```python
from build123d import *

# Parameters (mm, degrees)
SKETCH_W      = 45
SKETCH_H      = 161
PAD_DEPTH     = 10
SKETCH001_W   = 45
SKETCH001_H   = 10
PAD001_DEPTH  = 55.5
SKETCH002_R   = 2.75
HOLE_DEPTH    = 161.001
SKETCH003_W   = 45
SKETCH003_H   = 10
PAD002_DEPTH  = 45.4
SKETCH004_R   = 1.7
HOLE001_DEPTH = 10.001
SKETCH005_W   = 45
SKETCH005_H   = 10
PAD003_DEPTH  = 45
SKETCH006_R   = 1.7
HOLE002_DEPTH = 10.001
SKETCH007_R   = 10.125
SKETCH007_R_2 = 1.75
PAD004_DEPTH  = 3
SKETCH008_W   = 15
SKETCH008_H   = 4
PAD005_DEPTH  = 60
SKETCH009_R   = 19.35
SKETCH009_R_2 = 10.125
SKETCH009_R_3 = 1.75
PAD006_DEPTH  = 3
SKETCH010_W   = 12
SKETCH010_H   = 4
POCKET_DEPTH  = 8
FILLET_R      = 5


with BuildPart() as part:
    # Sketch → Pad (new body)
    with BuildSketch(Plane.XZ):
        with Locations((-22.5, 80.5)):
            Rectangle(SKETCH_W, SKETCH_H)
    extrude(amount=PAD_DEPTH)

    # Sketch001 (on Face6 of Pad) → Pad001 (join)
    with BuildSketch(Plane.XZ.offset(10)):
        with Locations((-22.5, 156)):
            Rectangle(SKETCH001_W, SKETCH001_H)
        with Locations((-22.5, 5)):
            Rectangle(SKETCH001_W, SKETCH001_H)
    extrude(amount=PAD001_DEPTH)

    # Sketch002 (on Face9 of Pad001) → Hole (cut, through all)
    with BuildSketch(Plane(origin=(0, 0, 161), x_dir=(-1, 0, 0), z_dir=(0, 0, 1))):
        with Locations((7.5, 59)):
            Circle(SKETCH002_R)
        with Locations((37.5, 59)):
            Circle(SKETCH002_R)
        with Locations((7.5, 27)):
            Circle(SKETCH002_R)
        with Locations((37.5, 27)):
            Circle(SKETCH002_R)
    extrude(amount=-HOLE_DEPTH, mode=Mode.SUBTRACT)

    # Sketch003 (on Face3 of Hole) → Pad002 (join)
    with BuildSketch(Plane(origin=(0, 0, 161), x_dir=(-1, 0, 0), z_dir=(0, 0, 1))):
        with Locations((22.5, 5)):
            Rectangle(SKETCH003_W, SKETCH003_H)
    extrude(amount=PAD002_DEPTH)

    # Sketch004 (on Face12 of Pad002) → Hole001 (cut, through all)
    with BuildSketch(Plane.XZ.offset(10)):
        with Locations((-32.5, 193.7)):
            Circle(SKETCH004_R)
        with Locations((-12.5, 193.7)):
            Circle(SKETCH004_R)
        with Locations((-32.5, 173.7)):
            Circle(SKETCH004_R)
        with Locations((-12.5, 173.7)):
            Circle(SKETCH004_R)
    extrude(amount=-HOLE001_DEPTH, mode=Mode.SUBTRACT)

    # Sketch005 (on Face16 of Hole001) → Pad003 (join)
    with BuildSketch(Plane(origin=(0, 0, 0), x_dir=(1, 0, 0), z_dir=(0, 0, -1))):
        with Locations((-22.5, 5)):
            Rectangle(SKETCH005_W, SKETCH005_H)
    extrude(amount=PAD003_DEPTH)

    # Sketch006 (on Face22 of Pad003) → Hole002 (cut, through all)
    with BuildSketch(Plane.XZ.offset(10)):
        with Locations((-32.5, -12.3)):
            Circle(SKETCH006_R)
        with Locations((-12.5, -12.3)):
            Circle(SKETCH006_R)
        with Locations((-32.5, -32.3)):
            Circle(SKETCH006_R)
        with Locations((-12.5, -32.3)):
            Circle(SKETCH006_R)
    extrude(amount=-HOLE002_DEPTH, mode=Mode.SUBTRACT)

    # Sketch007 (on Face2 of Hole002) → Pad004 (join)
    with BuildSketch(Plane(origin=(0, 37, 80), x_dir=(0, 0, -1), z_dir=(1, 0, 0))):
        with BuildLine():
            ThreePointArc((19.35, -3e-06), (0, 19.35), (-19.35, -3e-06))
            Line((-19.35, -3e-06), (-19.35, -37.000003))
            Line((-19.35, -37.000003), (19.35, -37.000003))
            Line((19.35, -37.000003), (19.35, -3e-06))
        make_face()
        Circle(SKETCH007_R, mode=Mode.SUBTRACT)
        with Locations((7.500003, 12.990379)):
            Circle(SKETCH007_R_2, mode=Mode.SUBTRACT)
        with Locations((-15, 5e-06)):
            Circle(SKETCH007_R_2, mode=Mode.SUBTRACT)
        with Locations((7.499994, -12.990384)):
            Circle(SKETCH007_R_2, mode=Mode.SUBTRACT)
    extrude(amount=-PAD004_DEPTH)

    # Sketch008 (on Face3 of Pad004) → Pad005 (join)
    with BuildSketch(Plane(origin=(-45, 0, 0), x_dir=(0, 0, -1), z_dir=(-1, 0, 0))):
        with Locations((-67.5, 2)):
            Rectangle(SKETCH008_W, SKETCH008_H)
    extrude(amount=PAD005_DEPTH)

    # Sketch009 (on Face25 of Pad005) → Pad006 (join)
    with BuildSketch(Plane(origin=(0, 0, 60), x_dir=(1, 0, 0), z_dir=(0, 0, -1))):
        with Locations((-114, -5)):
            Circle(SKETCH009_R)
        with Locations((-114, -5)):
            Circle(SKETCH009_R_2, mode=Mode.SUBTRACT)
        with Locations((-121.499999, 7.990382)):
            Circle(SKETCH009_R_3, mode=Mode.SUBTRACT)
        with Locations((-121.499999, -17.990382)):
            Circle(SKETCH009_R_3, mode=Mode.SUBTRACT)
        with Locations((-99, -5)):
            Circle(SKETCH009_R_3, mode=Mode.SUBTRACT)
    extrude(amount=-PAD006_DEPTH)

    # Sketch010 (on Face27 of Pad006) → Pocket (cut)
    with BuildSketch(Plane(origin=(0, 0, 75), x_dir=(-1, 0, 0), z_dir=(0, 0, 1))):
        with Locations((99, 2)):
            Rectangle(SKETCH010_W, SKETCH010_H)
    extrude(amount=-POCKET_DEPTH, mode=Mode.SUBTRACT)

    # Fillet
    fillet_edges = [part.edges().sort_by_distance(p)[0] for p in [
        (-45, -4, 67.5),
        (-3, -3e-06, 80),
    ]]
    fillet(fillet_edges, radius=FILLET_R)


solid = part.part
```
Check sheet for the modelled part. Datum: model origin and axes. Units: mm. A direction names the side the tool comes from. Round coordinates to 2 decimals unless told otherwise and drop trailing zeros. Order: outer loops, then holes, each group sorted by start corner. A loop starts at its lowest first (then second) coordinate and runs counter-clockwise, first axis right, second up.
1) Go/stop test with flat-tipped pins: pin 1 Ø4 at (x, z) = (-32.5, -12.3) entering from +Y; pin 2 Ø4.5 at (x, z) = (-12.5, 193.7) entering from -Y; pin 3 Ø9 at (x, y) = (-2, 10) entering from -Z. Record where each tip stops, or that it passes through.
2) Section check D-D (x = -17). Record the boundary of the cut face in (y, z).
3) Section check B-B (x = -37.5). Record the boundary of the cut face in (y, z), and give its area (3 significant figures).
4) Section check A-A (y = -27). Record the boundary of the cut face in (x, z).
5) Scan lines: line 1 (Y direction, x = -7, z = 158); line 2 (X direction, y = -3.75, z = 193.7); line 3 (X direction, y = -59, z = 5). Record each from-to range of solid material in increasing order.
6) Mould release check, pull along Y, two halves, no side actions. Record for faces 1 (the flat face through (-1, 17, 60.65)), 2 (the cylindrical face through (-7.142, -29.727, 5.07)), 3 (the flat face through (-23, -65.5, 156)): +Y half, -Y half, draft (parallel to the pull), parting line (faces both ways), or undercut.
7) Section check C-C (x = -111). Record the boundary of the cut face in (y, z).
8) Tool access check on faces 4 (the flat face through (-69, -2, 75)), 5 (the cylindrical face through (-47, -5, 67)), 6 (the flat face through (-23, -37, 161)), 7 (the flat face through (-23, -37, 10)). Record the directions out of +Z, -Z, +X, -X, +Y, -Y that give a thin tool (end or side, any length) a straight path to the whole face; none if there is none.
Result:
1. pin 1: stops at y = 0
1. pin 2: stops at y = -10
1. pin 3: stops at z = 60.65
2. outline: (-65.5, 0) - (-10, 0) - (-10, -45) - (0, -45) - (0, 206.4) - (-10, 206.4) - (-10, 161) - (-65.5, 161) - (-65.5, 151) - (-10, 151) - (-10, 10) - (-65.5, 10) - close
3. outline: (-65.5, 0) - (-61.75, 0) - (-61.75, 10) - (-65.5, 10) - close; (-65.5, 151) - (-61.75, 151) - (-61.75, 161) - (-65.5, 161) - close; (-56.25, 0) - (-29.75, 0) - (-29.75, 10) - (-56.25, 10) - close; (-56.25, 151) - (-29.75, 151) - (-29.75, 161) - (-56.25, 161) - close; (-24.25, 0) - (-10, 0) - (-10, -45) - (0, -45) - (0, 206.4) - (-10, 206.4) - (-10, 161) - (-24.25, 161) - (-24.25, 151) - (-10, 151) - (-10, 10) - (-24.25, 10) - close
3. area: 3,400 mm2
4. outline: (-45, 0) - (-40.25, 0) - (-40.25, 10) - (-45, 10) - close; (-45, 151) - (-40.25, 151) - (-40.25, 161) - (-45, 161) - close; (-34.75, 0) - (-10.25, 0) - (-10.25, 10) - (-34.75, 10) - close; (-34.75, 151) - (-10.25, 151) - (-10.25, 161) - (-34.75, 161) - close; (-4.75, 0) - (0, 0) - (0, 10) - (-4.75, 10) - close; (-4.75, 151) - (0, 151) - (0, 161) - (-4.75, 161) - close
5. line 1: y = -65.5 to -61.7, -56.3 to -29.7, -24.3 to 0
5. line 2: x = -45 to -34.2, -30.8 to -14.2, -10.8 to 0
5. line 3: x = -45 to -40.25, -34.75 to -10.25, -4.75 to 0
6. face 1: draft
6. face 2: undercut
6. face 3: -Y half
7. outline: (-14.12, 60) - (-4.67, 60) - (-4.67, 63) - (-14.12, 63) - close; (14.67, 60) - (24.12, 60) - (24.12, 63) - (14.67, 63) - close
8. face 4: +Z, -X, +Y, -Y
8. face 5: +Z, -Z, -Y
8. face 6: +Z, +X, -X, -Y
8. face 7: +X, -X, -Y
